Here's how the part is built. I have some questions about the finished solid (model axes, mm). Give positions to 0.01 mm unless a question says otherwise; leave off trailing zeros. Order: outer loops, then holes, each group sorted by start corner. A loop starts at its lowest first (then second) coordinate and runs counter-clockwise, first axis right, second up.
from build123d import *

# Parameters (mm, degrees)
SKETCH1_R           = 1.6
BOSS_EXTRUDE1_DEPTH = 3
FILLET1_R           = 5
SKETCH2_W           = 400
SKETCH2_H           = 15
CUT_EXTRUDE1_DEPTH  = 406.25794255
FILLET2_R           = 5
SKETCH3_W           = 45.5
SKETCH3_H           = 10
BOSS_EXTRUDE2_DEPTH = 3
FILLET3_R           = 5
SKETCH4_W           = 3.7
SKETCH4_H           = 15
CUT_EXTRUDE2_DEPTH  = 406.25794255


with BuildPart() as part:
    # Sketch1 → Boss-Extrude1 (new body)
    with BuildSketch(Plane(origin=(0, 0, 0), x_dir=(1, 0, 0), z_dir=(0, 1, 0))):
        Polygon((0, -15), (49.2, -15), (49.2, 0), (350.8, 0), (350.8, -15), (400, -15), (400, 30), (350.8, 30), (350.8, 65), (335.8, 65), (335.8, 15), (64.2, 15), (64.2, 65), (49.2, 65), (49.2, 30), (0, 30), align=None)
        with Locations(Location((9.6, 7.5, 0), (0, 0, 270))):
            Circle(SKETCH1_R, mode=Mode.SUBTRACT)
        with Locations(Location((39.6, 7.5, 0), (0, 0, 270))):
            Circle(SKETCH1_R, mode=Mode.SUBTRACT)
        with Locations(Location((39.6, -4, 0), (0, 0, 270))):
            Circle(SKETCH1_R, mode=Mode.SUBTRACT)
        with Locations(Location((9.6, -4, 0), (0, 0, 270))):
            Circle(SKETCH1_R, mode=Mode.SUBTRACT)
        with Locations(Location((343.3, 7.5, 0), (0, 0, 270))):
            Circle(SKETCH1_R, mode=Mode.SUBTRACT)
        with Locations(Location((56.7, 7.5, 0), (0, 0, 270))):
            Circle(SKETCH1_R, mode=Mode.SUBTRACT)
        with Locations(Location((81.7, 7.5, 0), (0, 0, 270))):
            Circle(SKETCH1_R, mode=Mode.SUBTRACT)
        with Locations(Location((106.7, 7.5, 0), (0, 0, 270))):
            Circle(SKETCH1_R, mode=Mode.SUBTRACT)
        with Locations(Location((131.7, 7.5, 0), (0, 0, 270))):
            Circle(SKETCH1_R, mode=Mode.SUBTRACT)
        with Locations(Location((156.7, 7.5, 0), (0, 0, 270))):
            Circle(SKETCH1_R, mode=Mode.SUBTRACT)
        with Locations(Location((243.3, 7.5, 0), (0, 0, 270))):
            Circle(SKETCH1_R, mode=Mode.SUBTRACT)
        with Locations(Location((268.3, 7.5, 0), (0, 0, 270))):
            Circle(SKETCH1_R, mode=Mode.SUBTRACT)
        with Locations(Location((293.3, 7.5, 0), (0, 0, 270))):
            Circle(SKETCH1_R, mode=Mode.SUBTRACT)
        with Locations(Location((318.3, 7.5, 0), (0, 0, 270))):
            Circle(SKETCH1_R, mode=Mode.SUBTRACT)
        with Locations(Location((39.6, 19, 0), (0, 0, 270))):
            Circle(SKETCH1_R, mode=Mode.SUBTRACT)
        with Locations(Location((9.6, 19, 0), (0, 0, 270))):
            Circle(SKETCH1_R, mode=Mode.SUBTRACT)
        with Locations(Location((390.4, 7.5, 0), (0, 0, 270))):
            Circle(SKETCH1_R, mode=Mode.SUBTRACT)
        with Locations(Location((360.4, 7.5, 0), (0, 0, 270))):
            Circle(SKETCH1_R, mode=Mode.SUBTRACT)
        with Locations(Location((390.4, -4, 0), (0, 0, 270))):
            Circle(SKETCH1_R, mode=Mode.SUBTRACT)
        with Locations(Location((360.4, -4, 0), (0, 0, 270))):
            Circle(SKETCH1_R, mode=Mode.SUBTRACT)
        with Locations(Location((56.7, 45, 0), (0, 0, 270))):
            Circle(SKETCH1_R, mode=Mode.SUBTRACT)
        with Locations(Location((56.7, 55, 0), (0, 0, 270))):
            Circle(SKETCH1_R, mode=Mode.SUBTRACT)
        with Locations(Location((390.4, 19, 0), (0, 0, 270))):
            Circle(SKETCH1_R, mode=Mode.SUBTRACT)
        with Locations(Location((360.4, 19, 0), (0, 0, 270))):
            Circle(SKETCH1_R, mode=Mode.SUBTRACT)
        with Locations(Location((343.3, 45, 0), (0, 0, 270))):
            Circle(SKETCH1_R, mode=Mode.SUBTRACT)
        with Locations(Location((343.3, 55, 0), (0, 0, 270))):
            Circle(SKETCH1_R, mode=Mode.SUBTRACT)
    extrude(amount=BOSS_EXTRUDE1_DEPTH)

    # Fillet1
    fillet1_edges = [part.edges().sort_by_distance(p)[0] for p in [
        (400, 1.5, 15),
        (350.8, 1.5, 15),
        (49.2, 1.5, 15),
        (0, 1.5, 15),
        (49.2, 1.5, -65),
        (64.2, 1.5, -65),
        (64.2, 1.5, -15),
        (335.8, 1.5, -15),
        (335.8, 1.5, -65),
        (350.8, 1.5, -65),
    ]]
    fillet(fillet1_edges, radius=FILLET1_R)

    # Sketch2 → Cut-Extrude1 (cut, through all)
    with BuildSketch(Plane(origin=(0, 3, 0), x_dir=(1, 0, 0), z_dir=(0, 1, 0))):
        with Locations((200, -7.5)):
            Rectangle(SKETCH2_W, SKETCH2_H)
    extrude(amount=-CUT_EXTRUDE1_DEPTH, mode=Mode.SUBTRACT)

    # Fillet2
    fillet2_edges = [part.edges().sort_by_distance(p)[0] for p in [
        (0, 1.5, 0),
        (400, 1.5, 0),
    ]]
    fillet(fillet2_edges, radius=FILLET2_R)

    # Sketch3 → Boss-Extrude2 (add)
    with BuildSketch(Plane.XZ):
        with Locations((377.25, -35)):
            Rectangle(SKETCH3_W, SKETCH3_H)
        with Locations((22.75, -35)):
            Rectangle(SKETCH3_W, SKETCH3_H)
    extrude(amount=-BOSS_EXTRUDE2_DEPTH)

    # Fillet3
    fillet3_edges = [part.edges().sort_by_distance(p)[0] for p in [
        (400, 1.5, -40),
        (354.5, 1.5, -40),
        (0, 1.5, -40),
        (45.5, 1.5, -40),
    ]]
    fillet(fillet3_edges, radius=FILLET3_R)

    # Sketch4 → Cut-Extrude2 (cut, through all)
    with BuildSketch(Plane(origin=(0, 3, 0), x_dir=(1, 0, 0), z_dir=(0, 1, 0))):
        with Locations((352.65, 22.5)):
            Rectangle(SKETCH4_W, SKETCH4_H)
        with Locations((47.35, 22.5)):
            Rectangle(SKETCH4_W, SKETCH4_H)
    extrude(amount=-CUT_EXTRUDE2_DEPTH, mode=Mode.SUBTRACT)


solid = part.part
Q1. I'm going to push flat-ended pins straight in: P1, Ø1.5, axis at x = 49.5, y = 0.5, coming from the -Z side; P2, Ø1.5, axis at x = 353.5, y = 1, coming from the -Z side; P3, Ø0.9, axis at x = 16.5, y = 1, coming from the -Z side. Where does each tip first touch, or does it pass through?
Filled sheet:
P1: stops at z = -63.07
P2: stops at z = -15
P3: stops at z = -40
Q2. I need wall thicknesses on L1, parallel to X at y = 2.4, z = -45; L2, parallel to X at y = 2.4, z = -28; L3, parallel to Z at x = 131.7, y = 1.65. Which ranges of each line are inside material? Lowest first, please.
Filled sheet:
L1: x = 49.2 to 55.1, 58.3 to 64.2, 335.8 to 341.7, 344.9 to 350.8
L2: x = 0 to 45.5, 49.2 to 64.2, 335.8 to 350.8, 354.5 to 400
L3: z = -15 to -9.1, -5.9 to 0
Q3. If we section it at B-B on x = 138.5: List the corners of the cut face in (y, z) for me.
Filled sheet:
outline: (0, -15) - (3, -15) - (3, 0) - (0, 0) - close
Q4. If we section it at A-A on z = -29: List the corners of the cut face in (x, y) for me, plus the area to 3 significant figures.
Filled sheet:
outline: (0, 0) - (45.5, 0) - (45.5, 3) - (0, 3) - close; (49.2, 0) - (64.2, 0) - (64.2, 3) - (49.2, 3) - close; (335.8, 0) - (350.8, 0) - (350.8, 3) - (335.8, 3) - close; (354.5, 0) - (400, 0) - (400, 3) - (354.5, 3) - close
area: 363 mm2
Q5. If we section it at C-C on y = 0.9: Give the number of separate pieces and of enclosed holes in the cut face, plus the area to 3 significant figures.
Filled sheet:
separate pieces: 1
enclosed holes: 22
area: 9,560 mm2
